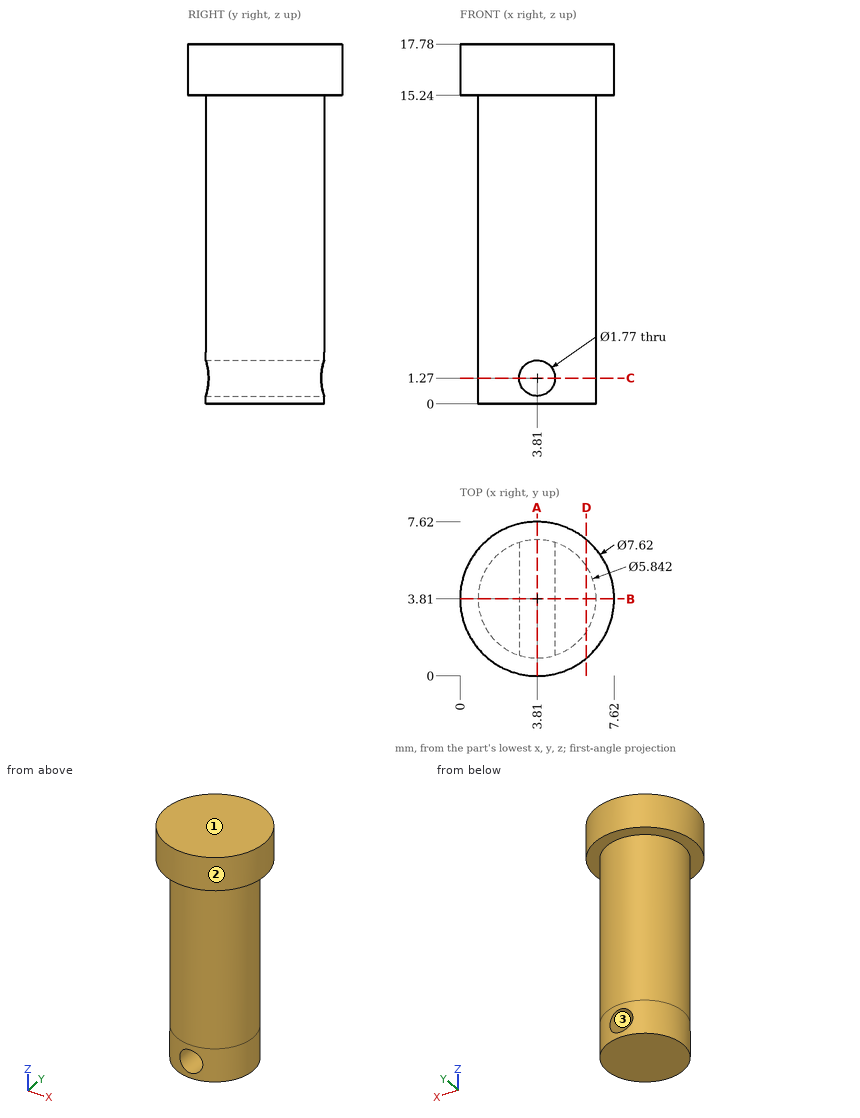
Design review of the part shown in the three views and the two pictorial views. Dimensions are in mm from the part's minimum x, y and z. Coordinates: 2 decimals unless noted, no trailing zeros. Write each loop counter-clockwise with the first axis right and the second up, starting at its lowest first coordinate (ties: lowest second). Pieces come first, ordered by that corner, then holes.
1) Clearance check with flat-ended pins moving along their axes: pin 1 Ø2.5 at (x, z) = (3.81, 1.27) entering from -Y; pin 2 Ø1 at (y, z) = (1.5, 4) entering from +X; pin 3 Ø2 at (y, z) = (3, 13) entering from -X. State where each tip first meets the part, or that it passes through.
2) To check wall thickness, follow probe 1 along Z at (x, y) = (3.81, 2.7) (3 decimals); probe 2 along Z at (x, y) = (4, 3); probe 3 along X at (y, z) = (1.25, 11.5). State the ranges of each line that lie inside material, in increasing order.
3) We need section C-C on z = 1.27. State the section outline as (x, y) points (3 decimals), then the cut area to 3 significant figures.
4) The part is to be moulded in two halves that separate along X. For the marked faces 1, 2 and 3, say which applies: pulls with the +X half, pulls with the -X half, needs draft (parallel to the pull), parting line crosses it, or undercut.
5) We need section A-A on x = 3.81. State the section outline as (y, z) points (3 decimals).
6) We need section D-D on x = 6.25. State the section outline as (y, z) points, then the cut area to 3 significant figures.
7) We need section B-B on y = 3.81. State the section outline as (x, z) points (3 decimals), then the cut area to 3 significant figures.
Answer list:
1. pin 1: stops at y = 0.89
1. pin 2: stops at x = 6.1
1. pin 3: stops at x = 0.89
2. probe 1: z = 0 to 0.385, 2.155 to 17.78
2. probe 2: z = 0 to 0.41, 2.13 to 17.78
2. probe 3: x = 2.4 to 5.22
3. outline: (2.925, 1.026) - (2.925, 6.594) arc R2.921 ccw to start; (4.695, 1.026) arc R2.921 ccw to (4.695, 6.594) - close
3. area: 16.6 mm2
4. face 1: needs draft
4. face 2: parting line crosses it
4. face 3: undercut
5. outline: (0, 15.24) - (0.889, 15.24) - (0.889, 2.155) - (6.731, 2.155) - (6.731, 15.24) - (7.62, 15.24) - (7.62, 17.78) - (0, 17.78) - close; (0.889, 0) - (6.731, 0) - (6.731, 0.385) - (0.889, 0.385) - close
6. outline: (0.88, 15.24) - (2.2, 15.24) - (2.2, 0) - (5.42, 0) - (5.42, 15.24) - (6.74, 15.24) - (6.74, 17.78) - (0.88, 17.78) - close
6. area: 63.8 mm2
7. outline: (0, 15.24) - (0.889, 15.24) - (0.889, 0) - (6.731, 0) - (6.731, 15.24) - (7.62, 15.24) - (7.62, 17.78) - (0, 17.78) - close; hole circle Ø1.77 at (3.81, 1.27)
7. area: 106 mm2
